from build123d import *

# Parameters (mm, degrees)
F2_DEPTH = 25
F3_DEPTH = 25


with BuildPart() as f2:
    # F1 (on Right) → F2 (new body, symmetric)
    with BuildSketch(Plane.YZ):
        with BuildLine():
            ThreePointArc((-89.915201, -9.228394), (-90.622307, -8.935501), (-90.915201, -8.228394))
            Line((-90.915201, -8.228394), (-90.915201, 87.817343))
            Line((-90.915201, 87.817343), (-93.915201, 87.817343))
            Line((-93.915201, 87.817343), (-93.915201, -9.228394))
            ThreePointArc((-93.915201, -9.228394), (-93.036521, -11.349715), (-90.915201, -12.228394))
            Line((-90.915201, -12.228394), (-13.896061, -12.228394))
            ThreePointArc((-13.896061, -12.228394), (-12.328566, -11.786315), (-11.223042, -10.590366))
            Line((-11.223042, -10.590366), (21.084799, 52.817343))
            Line((21.084799, 52.817343), (21.084799, 87.817343))
            Line((21.084799, 87.817343), (18.084799, 87.817343))
            Line((18.084799, 87.817343), (18.084799, 52.817343))
            Line((18.084799, 52.817343), (-13.250877, -8.682385))
            ThreePointArc((-13.250877, -8.682385), (-13.619385, -9.081035), (-14.141883, -9.228394))
            Line((-14.141883, -9.228394), (-89.915201, -9.228394))
        make_face()
    extrude(amount=F2_DEPTH, both=True)

    # F0 (on Front) → F3 (cut)
    with BuildSketch(Plane.XZ):
        with BuildLine():
            ThreePointArc((-9, 66.817343), (0, 57.817343), (9, 66.817343))
            ThreePointArc((9, 66.817343), (0, 75.817343), (-9, 66.817343))
        make_face()
        with BuildLine():
            Line((9, 66.817343), (9, 87.817343))
            Line((9, 87.817343), (-9, 87.817343))
            Line((-9, 87.817343), (-9, 66.817343))
            ThreePointArc((-9, 66.817343), (0, 75.817343), (9, 66.817343))
        make_face()
    extrude(amount=-F3_DEPTH, mode=Mode.SUBTRACT)


solid = f2.part
Read the model definition and answer for the solid it produces. Units are mm, in the model's axes. A direction names the side the tool comes from. Round coordinates to 2 decimals unless told otherwise and drop trailing zeros. Order: outer loops, then holes, each group sorted by start corner. A loop starts at its lowest first (then second) coordinate and runs counter-clockwise, first axis right, second up.
1) The part is cut by section B-B on x = 0. Write down the section's boundary in (y, z).
2) The part is cut by section D-D on y = -74. Write down the section's boundary in (x, z).
3) For faces 1 (the face through (-0.2, 19.56, 57.82)), 2 (the face through (0.35, 4.705, 20.67)), 3 (the face through (0, -51, -9.228)), determine the directions among +Z, -Z, +X, -X, +Y, -Y from which every point of the face is accessible in a straight line to the end or side of a thin tool.
4) The part is cut by section C-C on z = 29. Write down the section's boundary in (x, y), plus the area to 3 significant figures.
5) Flat-ended cylindrical pins translate along their axes: pin 1 (15 mm diameter, centred on x = 9.5, y = -55.5, fed in from +Z); pin 2 (5 mm diameter, centred on x = 2, z = 75.5, fed in from +Y); pin 3 (12 mm diameter, centred on x = 13.5, z = 42.5, fed in from +Y) (3 decimals). Find the tip coordinate at first contact, or state that the pin passes through.
6) The part is cut by section A-A on z = 70. Write down the section's boundary in (x, y).
7) Straight lines are drawn through the part: L1, parallel to Y at x = -11.5, z = 58.5; L2, parallel to Z at x = 6, y = -42; L3, parallel to Y at x = -9, z = 40. For each, find the intervals that lie inside material, in ascending order.
8) The mould has two halves that part along X. Classify faces 4 (the face through (25, -45, -10)), 5 (the face through (11, 21.085, 70)), 6 (the face through (-9, 20, 77)), 7 (the face through (-25, -45, -10)): released by +X, released by -X, zero draft, split by the parting line, or undercut.
Resolved:
1. outline: (-93.92, -9.23) arc R3 ccw to (-90.92, -12.23) - (-13.9, -12.23) arc R3 ccw to (-11.22, -10.59) - (21.08, 52.82) - (21.08, 57.82) - (18.08, 57.82) - (18.08, 52.82) - (-13.25, -8.68) arc R1 cw to (-14.14, -9.23) - (-89.92, -9.23) arc R1 cw to (-90.92, -8.23) - (-90.92, 87.82) - (-93.92, 87.82) - close
2. outline: (-25, -12.23) - (25, -12.23) - (25, -9.23) - (-25, -9.23) - close
3. face 1: +Z, +Y
3. face 2: -Z, +X, -X, +Y
3. face 3: +Z, +X, -X
4. outline: (-25, -93.92) - (25, -93.92) - (25, -90.92) - (-25, -90.92) - close; (-25, 5.95) - (25, 5.95) - (25, 8.95) - (-25, 8.95) - close
4. area: 300 mm2
5. pin 1: stops at z = -9.23
5. pin 2: stops at y = -90.92
5. pin 3: stops at y = 18.885
6. outline: (-25, -93.92) - (25, -93.92) - (25, -90.92) - (-25, -90.92) - close; (-25, 18.08) - (-9, 18.08) - (-9, 21.08) - (-25, 21.08) - close; (9, 18.08) - (25, 18.08) - (25, 21.08) - (9, 21.08) - close
7. L1: y = -93.92 to -90.92, 18.08 to 21.08
7. L2: z = -12.23 to -9.23
7. L3: y = -93.92 to -90.92, 11.55 to 14.55
8. face 4: released by +X
8. face 5: zero draft
8. face 6: undercut
8. face 7: released by -X
